from build123d import *

# Parameters (mm, degrees)
SKETCH1_W                           = 23
SKETCH1_H                           = 15
BOSS_EXTRUDE1_DEPTH                 = 3
BOSS_EXTRUDE2_DEPTH                 = 12.5
BOSS_EXTRUDE2_DEPTH_BACK            = 3
SKETCH2_W                           = 3
SKETCH2_H                           = 15
BOSS_EXTRUDE3_DEPTH                 = 10
TAP_START                           = -2.5
TAP_DRILL_FOR_M2X0_4_TAP1_OUTLINE_R = 0.8
TAP_DRILL_FOR_M2X0_4_TAP1_DEPTH     = 10
SKETCH6_W                           = 29
SKETCH6_H                           = 20
BOSS_EXTRUDE4_DEPTH                 = 3
SKETCH7_W                           = 10
SKETCH7_H                           = 10
CUT_EXTRUDE1_DEPTH                  = 35.301056835
CUT_EXTRUDE2_DEPTH                  = 2
F_4_0_4_DIAMETER_HOLE1_D            = 4
F_4_0_4_DIAMETER_HOLE1_DEPTH        = 10
F_4_0_4_DIAMETER_HOLE1_TIP          = 1.201721238
SKETCH12_W                          = 29
SKETCH12_H                          = 15
BOSS_EXTRUDE5_DEPTH                 = 2
SKETCH13_W                          = 3
SKETCH13_H                          = 7
CUT_EXTRUDE4_DEPTH                  = 3.5
CHAMFER1_SIZE                       = 2
FILLET1_R                           = 5


# Read off the part's stored shape, not the designer's step: Tap Drill for M2x0.4 Tap1
with BuildPart() as part:
    # Sketch1 → Boss-Extrude1 (new body)
    with BuildSketch(Plane(origin=(0, 0, 0), x_dir=(1, 0, 0), z_dir=(0, 1, 0))):
        Rectangle(SKETCH1_W, SKETCH1_H)
    extrude(amount=BOSS_EXTRUDE1_DEPTH)

    # Sketch2 → Boss-Extrude2 (add, two sides: drawn at the far end of the back side and taken through both)
    with BuildSketch(Plane(origin=(0, 3, 0), x_dir=(1, 0, 0), z_dir=(0, 1, 0)).offset(-BOSS_EXTRUDE2_DEPTH_BACK)):
        with Locations((13, 0)):
            Rectangle(SKETCH2_W, SKETCH2_H)
        with Locations((-13, 0)):
            Rectangle(SKETCH2_W, SKETCH2_H)
    extrude(amount=BOSS_EXTRUDE2_DEPTH + BOSS_EXTRUDE2_DEPTH_BACK)

    # Sketch3 → Boss-Extrude3 (add)
    with BuildSketch(Plane.XY.offset(7.5)):
        with BuildLine():
            ThreePointArc((16.25, 9.5), (15.765564437, 10.979019946), (14.5, 11.884848004))
            Line((14.5, 11.884848004), (14.5, 7.115151996))
            ThreePointArc((14.5, 7.115151996), (15.765564437, 8.020980054), (16.25, 9.5))
        make_face()
        with BuildLine():
            Line((-14.5, 7.115151996), (-14.5, 11.884848004))
            ThreePointArc((-14.5, 11.884848004), (-16.25, 9.5), (-14.5, 7.115151996))
        make_face()
    extrude(amount=-BOSS_EXTRUDE3_DEPTH)

    # Tap Drill for M2x0.4 Tap1 outline → Tap Drill for M2x0.4 Tap1 (cut)
    with BuildSketch(Plane.XY.offset(TAP_START)):
        with Locations((-13.75, 9.5)):
            Circle(TAP_DRILL_FOR_M2X0_4_TAP1_OUTLINE_R)
    extrude(amount=TAP_DRILL_FOR_M2X0_4_TAP1_DEPTH, mode=Mode.SUBTRACT)

    # Tap Drill for M2x0.4 Tap1 2 outline → Tap Drill for M2x0.4 Tap1 2 (revolve, cut)
    with BuildSketch(Plane(origin=(13.75, 9.5, 0), x_dir=(1, 0, 0), z_dir=(0, -1, 0))):
        Polygon((0, 7.5), (0, -2.980688495), (0.800001695, -2.499998981), (0.8, 7.5), align=None)
    revolve(axis=Axis((13.75, 9.5, 0), (0, 0, 1)), mode=Mode.SUBTRACT)

    # Sketch6 → Boss-Extrude4 (add)
    with BuildSketch(Plane.XZ):
        with Locations((0, 17.5)):
            Rectangle(SKETCH6_W, SKETCH6_H)
    extrude(amount=-BOSS_EXTRUDE4_DEPTH)

    # Sketch7 → Cut-Extrude1 (cut, through all)
    with BuildSketch(Plane(origin=(0, 3, 0), x_dir=(1, 0, 0), z_dir=(0, 1, 0))):
        with Locations((9.5, -22.5)):
            Rectangle(SKETCH7_W, SKETCH7_H)
    extrude(amount=-CUT_EXTRUDE1_DEPTH, mode=Mode.SUBTRACT)

    # Sketch8 → Cut-Extrude2 (cut)
    with BuildSketch(Plane.XZ.offset(-3)):
        Polygon((-5.767949192, 17), (-4.035898385, 20), (-5.767949192, 23), (-9.232050808, 23), (-10.964101615, 20), (-9.232050808, 17), align=None)
    extrude(amount=CUT_EXTRUDE2_DEPTH, mode=Mode.SUBTRACT)

    # Ø4.0 (4) Diameter Hole1
    with Locations(Plane(origin=(0, 0, 0), x_dir=(-1, 0, 0), z_dir=(0, -1, 0))):
        with Locations((7.5, -20)):
            Hole(F_4_0_4_DIAMETER_HOLE1_D / 2, depth=F_4_0_4_DIAMETER_HOLE1_DEPTH)
            with Locations((0, 0, -(F_4_0_4_DIAMETER_HOLE1_DEPTH + F_4_0_4_DIAMETER_HOLE1_TIP / 2))):  # 118° drill point
                Cone(0, F_4_0_4_DIAMETER_HOLE1_D / 2, F_4_0_4_DIAMETER_HOLE1_TIP, mode=Mode.SUBTRACT)

    # Sketch12 → Boss-Extrude5 (add)
    with BuildSketch(Plane(origin=(0, 15.5, 0), x_dir=(1, 0, 0), z_dir=(0, 1, 0))):
        Rectangle(SKETCH12_W, SKETCH12_H)
    extrude(amount=BOSS_EXTRUDE5_DEPTH)

    # Sketch13 → Cut-Extrude4 (cut)
    with BuildSketch(Plane(origin=(0, 0, -7.5), x_dir=(-1, 0, 0), z_dir=(0, 0, -1))):
        with Locations((-13, 9.25)):
            Rectangle(SKETCH13_W, SKETCH13_H)
    extrude(amount=-CUT_EXTRUDE4_DEPTH, mode=Mode.SUBTRACT)

    # Chamfer1
    chamfer1_edges = [part.edges().sort_by_distance(p)[0] for p in [
        (-14.5, 17.5, 0),
        (14.5, 17.5, 0),
    ]]
    chamfer(chamfer1_edges, length=CHAMFER1_SIZE)

    # Fillet1
    # the kernel refuses this fillet: 5 mm, written as the material it takes off along each edge
    with BuildSketch(Plane(origin=(-14.5, -12.5, 27.5), x_dir=(0, 0, -1), z_dir=(0, 1, 0))) as fillet1_piece_1:
        with BuildLine():
            CenterArc((FILLET1_R, -FILLET1_R), FILLET1_R, 90, 90)
            Line((0, -FILLET1_R), (0, 0))
            Line((0, 0), (FILLET1_R, 0))
        make_face()
    extrude(amount=28, mode=Mode.SUBTRACT)
    with BuildSketch(Plane(origin=(-14.5, 28, -7.5), x_dir=(0, 0, 1), z_dir=(0, -1, 0))) as fillet1_piece_2:
        with BuildLine():
            CenterArc((FILLET1_R, -FILLET1_R), FILLET1_R, 90, 90)
            Line((0, -FILLET1_R), (0, 0))
            Line((0, 0), (FILLET1_R, 0))
        make_face()
    extrude(amount=40.5, mode=Mode.SUBTRACT)


solid = part.part
Work out the finished part from the listing and answer in its coordinate system (mm). A direction names the side the tool comes from. Give positions to 0.01 mm unless a question says otherwise; leave off trailing zeros. Order: outer loops, then holes, each group sorted by start corner. A loop starts at its lowest first (then second) coordinate and runs counter-clockwise, first axis right, second up. Notation, with made-up numbers: (29, 1) -> (36, 1) arc R18 cw to (36, 33) -> close; hole circle Ø8 at (31.25, -25). An arc over 180 degrees is marked (long way). One line per item, written item: value.
Item 1: Find section A-A, the plane z = 6. Give the vertices of the cut face in (x, y), plus the area to 3 significant figures.
Answer sheet:
outline: (-14.5, 0) -> (14.5, 0) -> (14.5, 7.12) arc R2.5 ccw to (14.5, 11.88) -> (14.5, 15.5) -> (12.5, 17.5) -> (-12.5, 17.5) -> (-14.5, 15.5) -> (-14.5, 11.88) arc R2.5 ccw to (-14.5, 7.12) -> close; hole circle Ø1.6 at (-13.75, 9.5); hole (-11.5, 3) -> (11.5, 3) -> (11.5, 15.5) -> (-11.5, 15.5) -> close; hole circle Ø1.6 at (13.75, 9.5)
area: 224 mm²
Item 2: Find section C-C, the plane x = -7.5. Give the vertices of the cut face in (y, z), plus the area to 3 significant figures.
Answer sheet:
outline: (0, -7.5) -> (3, -7.5) -> (3, 17) -> (1, 17) -> (1, 18) -> (0, 18) -> close; (0, 22) -> (1, 22) -> (1, 23) -> (3, 23) -> (3, 27.5) -> (0, 27.5) -> close; (15.5, -7.5) -> (17.5, -7.5) -> (17.5, 7.5) -> (15.5, 7.5) -> close
area: 119 mm²
Item 3: Flat-ended cylindrical pins translate along their axes: P1, Ø1.4, axis at x = 15, y = 10, coming from the -Z side; P2, Ø2, axis at y = 11.5, z = 2.5, coming from the -X side; P3, Ø8, axis at y = 2.5, z = 18.5, coming from the +X side; P4, Ø2, axis at x = 8, y = 5.5, coming from the -Z side. Find the tip coordinate at first contact, or state that the pin passes through.
Answer sheet:
P1: z = -4
P2: x = -16.04
P3: x = 14.5
P4: through
Item 4: Find section D-D, the plane x = 8. Give the vertices of the cut face in (y, z), plus the area to 3 significant figures.
Answer sheet:
outline: (0, -7.5) -> (3, -7.5) -> (3, 17.5) -> (0, 17.5) -> close; (15.5, -7.5) -> (17.5, -7.5) -> (17.5, 7.5) -> (15.5, 7.5) -> close
area: 105 mm²
Item 5: Determine the mould class of faces 4 (the cylindrical face through (-13.07, 1.48, 26)), 5 (the flat face through (-10.1, 2, 18.5)), 6 (the flat face through (13, 9, -4)) for opening direction Z: released by +Z, released by -Z, zero draft, split by the parting line, or undercut.
Answer sheet:
face 4: released by +Z
face 5: undercut
face 6: released by -Z
Item 6: A tool of negligible diameter and unlimited length cuts with its end or side. For faces 1 (the flat face through (13, 12.75, -6)), 2 (the flat face through (-14.5, 3, 7)), 3 (the flat face through (-6.78, 1, 22.04)), from which of +Z, -Z, +X, -X, +Y, -Y can it reach the whole face along a straight path? Write none if from no direction.
Answer sheet:
face 1: -Z, +X
face 2: +Z, -Z, -X, -Y
face 3: +Y
Item 7: Straight lines are drawn through the part: probe 1 along Y at (x, z) = (-4, 3.5); probe 2 along X at (y, z) = (0.35, 20); probe 3 along X at (y, z) = (3.5, -1). For each, find the intervals that lie inside material, in ascending order.
Answer sheet:
probe 1: 0 to 3, 15.5 to 17.5
probe 2: -14.5 to -9.5, -5.5 to 4.5
probe 3: -14.5 to -11.5, 11.5 to 14.5
Item 8: Find section B-B, the plane y = 14.25. Give the vertices of the cut face in (x, z).
Answer sheet:
outline: (-14.5, -2.5) arc R5 ccw to (-11.5, -7.08) -> (-11.5, 7.5) -> (-14.5, 7.5) -> close; (11.5, -7.5) -> (14.5, -7.5) -> (14.5, 7.5) -> (11.5, 7.5) -> close
